```python
from build123d import *

# Parameters (mm, degrees)
SKETCH1_R           = 28.321
SKETCH1_R_2         = 22.225
BOSS_EXTRUDE1_DEPTH = 10
SKETCH1_2_R         = 22.225
BOSS_EXTRUDE2_DEPTH = 70
SKETCH1_3_R         = 22.225
BOSS_EXTRUDE3_DEPTH = 10


with BuildPart() as part:
    # Sketch1 → Boss-Extrude1 (new body)
    with BuildSketch(Plane(origin=(0, 0, 0), x_dir=(1, 0, 0), z_dir=(0, 1, 0))):
        Circle(SKETCH1_R)
        Circle(SKETCH1_R_2, mode=Mode.SUBTRACT)
    extrude(amount=BOSS_EXTRUDE1_DEPTH)



with BuildPart() as body_2:
    # Sketch1<2> → Boss-Extrude2 (new body)
    with BuildSketch(Plane(origin=(0, 0, 0), x_dir=(1, 0, 0), z_dir=(0, 1, 0))):
        Circle(SKETCH1_2_R)
    extrude(amount=-BOSS_EXTRUDE2_DEPTH)


with BuildPart() as part_1:
    add(part.part)

    add(body_2.part)  # Boss-Extrude3 merges body 2
    # Sketch1<3> → Boss-Extrude3 (add)
    with BuildSketch(Plane(origin=(0, 0, 0), x_dir=(1, 0, 0), z_dir=(0, 1, 0))):
        Circle(SKETCH1_3_R)
    extrude(amount=BOSS_EXTRUDE3_DEPTH)


solid = part_1.part
```
The model under review builds one solid part; all positions refer to its coordinate system, in mm. A direction names the side the tool comes from. Round coordinates to 2 decimals unless told otherwise and drop trailing zeros. Order: outer loops, then holes, each group sorted by start corner. A loop starts at its lowest first (then second) coordinate and runs counter-clockwise, first axis right, second up. Notation, with made-up numbers: (44.5, 60.25) -> (59.5, 60.25) arc R18 cw to (59.5, 86.25) -> close; hole circle Ø11 at (10.25, -37.5). An arc over 180 degrees is marked (long way). Use a Markdown table: item, result.
Q1. Tool access review of faces 1 (the cylindrical face through (21.199, -34.51, -6.676)), 2 (the flat face through (0, -70, 0)): name each direction out of +Z, -Z, +X, -X, +Y, -Y from which nothing blocks a thin tool from reaching the whole face with its end or side.
Values:
| item | result |
|---|---|
| face 1 | -Y |
| face 2 | +Z, -Z, +X, -X, -Y |
Q2. For line 1 (Y direction, x = 18, z = -17); line 2 (Z direction, x = -8.5, y = -43); line 3 (Z direction, x = -5, y = -32.5), list the stretches that pass through material, from the lowest coordinate up.
Values:
| item | result |
|---|---|
| line 1 | y = 0 to 10 |
| line 2 | z = -20.54 to 20.54 |
| line 3 | z = -21.66 to 21.66 |
Q3. We need section A-A on z = 0. Write out the cut boundary in (x, y) (3 decimals), then the cut area to 3 significant figures.
Values:
| item | result |
|---|---|
| outline | (-28.321, 0) -> (-22.225, 0) -> (-22.225, -70) -> (22.225, -70) -> (22.225, 0) -> (28.321, 0) -> (28.321, 10) -> (-28.321, 10) -> close |
| area | 3,680 mm^2 |
Q4. We need section C-C on y = -40.5. Write out the cut boundary in (x, z) (3 decimals), then the cut area to 3 significant figures.
Values:
| item | result |
|---|---|
| outline | circle Ø44.45 at (0, 0) |
| area | 1,550 mm^2 |
Q5. Clearance check with flat-ended pins moving along their axes: P1, Ø2, axis at x = -16, z = 21, coming from the -Y side; P2, Ø1.5, axis at y = -58.5, z = -12, coming from the +X side; P3, Ø10, axis at y = -11, z = -5.5, coming from the -X side. State where each tip first meets the part, or that it passes through.
Values:
| item | result |
|---|---|
| P1 | stops at y = 0 |
| P2 | stops at x = 19.17 |
| P3 | stops at x = -22.22 |
Q6. We need section B-B on x = 0. Write out the cut boundary in (y, z) (3 decimals).
Values:
| item | result |
|---|---|
| outline | (-70, -22.225) -> (0, -22.225) -> (0, -28.321) -> (10, -28.321) -> (10, 28.321) -> (0, 28.321) -> (0, 22.225) -> (-70, 22.225) -> close |
